from build123d import *

# Parameters (mm, degrees)
F0_R     = 9.2551404176
F1_DEPTH = 25
F3_F1_R  = 5
F3_F2_R  = 5
F3_F3_R  = 5
F3_F4_R  = 5
F3_F5_R  = 5
F3_F6_R  = 5
F3_F7_R  = 5
F3_F8_R  = 5
F3_F9_R  = 5


# Not quite as in the source:
# - a feature of the source that left no trace in its solid (it failed there, or was rolled back) is left out


with BuildPart() as f1:
    # F0 (on Top) → F1 (new body)
    with BuildSketch(Plane.XY):
        with BuildLine():
            Line((50, -25), (50, 25))
            Line((50, 25), (-40, 25))
            ThreePointArc((-40, 25), (-42.9289321881, 17.9289321881), (-50, 15))
            Line((-50, 15), (-50, -25))
            Line((-50, -25), (50, -25))
        make_face()
        with Locations((26.5483168381, 0.0399786921)):
            Circle(F0_R, mode=Mode.SUBTRACT)
    extrude(amount=F1_DEPTH)

    # F3: fillet of radius 5 on 15 edges, made by hand

    # F3_f1
    f3_f1_edges = [f1.edges().sort_by_distance(p)[0] for p in [
        (-50, 15, 12.5),
    ]]
    fillet(f3_f1_edges, radius=F3_F1_R)

    # F3_f2
    f3_f2_edges = [f1.edges().sort_by_distance(p)[0] for p in [
        (-50, -25, 12.5),
    ]]
    fillet(f3_f2_edges, radius=F3_F2_R)

    # F3_f3
    f3_f3_edges = [f1.edges().sort_by_distance(p)[0] for p in [
        (50, -25, 12.5),
    ]]
    fillet(f3_f3_edges, radius=F3_F3_R)

    # F3_f4
    f3_f4_edges = [f1.edges().sort_by_distance(p)[0] for p in [
        (50, 25, 12.5),
    ]]
    fillet(f3_f4_edges, radius=F3_F4_R)

    # F3_f5
    f3_f5_edges = [f1.edges().sort_by_distance(p)[0] for p in [
        (-40, 25, 12.5),
    ]]
    fillet(f3_f5_edges, radius=F3_F5_R)

    # F3_f6
    f3_f6_edges = [f1.edges().sort_by_distance(p)[0] for p in [
        (-50, -4.5710678119, 0),
    ]]
    fillet(f3_f6_edges, radius=F3_F6_R)

    # F3_f7
    f3_f7_edges = [f1.edges().sort_by_distance(p)[0] for p in [
        (-50, -4.5710678119, 25),
    ]]
    fillet(f3_f7_edges, radius=F3_F7_R)

    # F3_f8
    f3_f8_edges = [f1.edges().sort_by_distance(p)[0] for p in [
        (17.2931764204, 0.0399786921, 0),
    ]]
    fillet(f3_f8_edges, radius=F3_F8_R)

    # F3_f9
    f3_f9_edges = [f1.edges().sort_by_distance(p)[0] for p in [
        (17.2931764204, 0.0399786921, 25),
    ]]
    fillet(f3_f9_edges, radius=F3_F9_R)


solid = f1.part
Design review of the part built by this model. Coordinates are the model's own, in mm. Coordinates: 2 decimals unless noted, no trailing zeros. Order: outer loops, then holes, each group sorted by start corner. A loop starts at its lowest first (then second) coordinate and runs counter-clockwise, first axis right, second up. Notation, with made-up numbers: (14.5, 55.25) -> (26.5, 55.25) arc R25 ccw to (26.5, 88.25) -> close; hole circle Ø9 at (60.25, 69.25). An arc over 180 degrees is marked (long way). One line per item, written item: value.
1) We need section A-A, the plane x = 3. Give the boundary of the cut face in (y, z).
Output values:
outline: (-25, 5) arc R5 ccw to (-20, 0) -> (20, 0) arc R5 ccw to (25, 5) -> (25, 20) arc R5 ccw to (20, 25) -> (-20, 25) arc R5 ccw to (-25, 20) -> close
2) To check wall thickness, follow probe 1 along Y at (x, z) = (27, 12); probe 2 along X at (y, z) = (-8, 2); probe 3 along X at (y, z) = (-6.5, 19.25). State the ranges of each line that lie inside material, in increasing order. Write a range as [from, to].
Output values:
probe 1: y = [-25, -9.2], [9.28, 25]
probe 2: x = [-49, 20.18], [32.91, 49]
probe 3: x = [-50, 20], [33.1, 50]
3) We need section B-B, the plane z = 11. Give the boundary of the cut face in (x, y), then the cut area to 3 significant figures.
Output values:
outline: (-50, -20) arc R5 ccw to (-45, -25) -> (45, -25) arc R5 ccw to (50, -20) -> (50, 20) arc R5 ccw to (45, 25) -> (-35.86, 25) arc R5 ccw to (-40.57, 21.67) arc R10 cw to (-46.67, 15.57) arc R5 ccw to (-50, 10.86) -> close; hole circle Ø18.51 at (26.55, 0.04)
area: 4,630 mm2
4) We need section C-C, the plane y = -21. Give the boundary of the cut face in (x, z), then the cut area to 3 significant figures.
Output values:
outline: (-49.9, 5) arc R4.9 ccw to (-45, 0.1) -> (45, 0.1) arc R4.9 ccw to (49.9, 5) -> (49.9, 20) arc R4.9 ccw to (45, 24.9) -> (-45, 24.9) arc R4.9 ccw to (-49.9, 20) -> close
area: 2,450 mm2
5) Clearance check with flat-ended pins moving along their axes: P1, Ø1.5, axis at y = -9, z = 22, coming from the +X side; P2, Ø3, axis at x = -38, z = 8, coming from the +Y side. State where each tip first meets the part, or that it passes through.
Output values:
P1: stops at x = 49.84
P2: stops at y = 24.96
